Source: CAD feature listing. Evaluate the final solid. Frame: model axes, mm. A direction names the side the tool comes from. Give positions to 0.01 mm unless a question says otherwise; leave off trailing zeros. Loops run counter-clockwise (first coordinate to the right, second up) from the corner with the lowest first, then second, coordinate; pieces in that order, holes last. Notation, with made-up numbers: M 68.5,-3 L 87.5,-3 A32 cw 87.5,28 Z; hole C -23,39 d11. An arc over 180 degrees is marked long. Answer in a Markdown table with one row per item.
```python
from build123d import *

# Parameters (mm, degrees)
BOSS_EXTRUDE1_DEPTH = 38.1
SKETCH2_W           = 31.75
SKETCH2_H           = 31.75
CUT_EXTRUDE1_DEPTH  = 73.334276799


with BuildPart() as part:
    # Sketch1 → Boss-Extrude1 (new body)
    with BuildSketch(Plane(origin=(0, 0, 0), x_dir=(0, 0, -1), z_dir=(1, 0, 0))):
        with BuildLine():
            Line((48.26, 38.1), (0, 38.1))
            Line((0, 38.1), (29.621235626, 0))
            Line((29.621235626, 0), (48.26, 0))
            ThreePointArc((48.26, 0), (38.940617813, 19.05), (48.26, 38.1))
        make_face()
    extrude(amount=BOSS_EXTRUDE1_DEPTH)

    # Sketch2 → Cut-Extrude1 (cut, through all)
    with BuildSketch(Plane.XY):
        with Locations((19.05, 19.05)):
            Rectangle(SKETCH2_W, SKETCH2_H)
    extrude(amount=-CUT_EXTRUDE1_DEPTH, mode=Mode.SUBTRACT)


solid = part.part
```
Q1. Section query A-A (z = -33). Output: boundary loops of the cut face in (x, y) (3 decimals), plus the area to 3 significant figures.
Values follow:
| item | result |
|---|---|
| outline | M 0,0 L 38.1,0 L 38.1,38.1 L 0,38.1 Z; hole M 3.175,3.175 L 34.925,3.175 L 34.925,34.925 L 3.175,34.925 Z |
| area | 444 mm^2 |
Q2. Ray query, probe 1 along Y at (x, z) = (25.5, -38) (3 decimals); probe 2 along Y at (x, z) = (21, -7.5) (3 decimals). Return the intervals inside material, ascending. Write a range as from..to.
Values follow:
| item | result |
|---|---|
| probe 1 | 0..3.175, 34.925..38.1 |
| probe 2 | 34.925..38.1 |
Q3. Section query C-C (y = 24). Output: boundary loops of the cut face in (x, z) (3 decimals), plus the area to 3 significant figures.
Values follow:
| item | result |
|---|---|
| outline | M 0,-39.454 L 3.175,-39.454 L 3.175,-10.962 L 0,-10.962 Z; M 34.925,-39.454 L 38.1,-39.454 L 38.1,-10.962 L 34.925,-10.962 Z |
| area | 181 mm^2 |
Q4. Mould query, pull axis X, two halves, no side actions, for faces 3 (the flat face through (3.175, 22, -28)), 4 (the flat face through (19, 0, -39)), 5 (the flat face through (38.1, 24, -29)). Classes: +X half, -X half, draft (parallel to the pull), parting line (faces both ways), or undercut.
Values follow:
| item | result |
|---|---|
| face 3 | undercut |
| face 4 | draft |
| face 5 | +X half |
Q5. Section query D-D (z = -18). Output: boundary loops of the cut face in (x, y) (3 decimals), plus the area to 3 significant figures.
Values follow:
| item | result |
|---|---|
| outline | M 0,14.948 L 3.175,14.948 L 3.175,34.925 L 34.925,34.925 L 34.925,14.948 L 38.1,14.948 L 38.1,38.1 L 0,38.1 Z |
| area | 248 mm^2 |
Q6. Contact query for flat-ended pins moving along their axis: pin 1 Ø4 at (x, z) = (13, -20) entering from -Y (3 decimals); pin 2 Ø10 at (y, z) = (25.5, -42) entering from -X. Output: stop coordinate, or through.
Values follow:
| item | result |
|---|---|
| pin 1 | y = 34.925 |
| pin 2 | x = 0 |
Q7. Reachability of faces 1 (the flat face through (34.925, 22, -28)), 2 (the flat face through (0, 24, -29)) from +Z, -Z, +X, -X, +Y, -Y: full face, straight path, thin tool, end or side. Return the list, or none.
Values follow:
| item | result |
|---|---|
| face 1 | +Z, -Z |
| face 2 | +Z, -Z, -X, +Y, -Y |
Q8. Section query B-B (x = 24.5). Output: boundary loops of the cut face in (y, z) (3 decimals), plus the area to 3 significant figures.
Values follow:
| item | result |
|---|---|
| outline | M 0,-48.26 A24.13 cw 3.175,-44.898 L 3.175,-27.153 L 0,-29.621 Z; M 34.925,-44.898 A24.13 cw 38.1,-48.26 L 38.1,0 L 34.925,-2.468 Z |
| area | 201 mm^2 |
